from build123d import *

# Parameters (mm, degrees)
F0_W     = 19.05
F0_H     = 177.8
F1_DEPTH = 19.05
F2_R     = 3.175
F3_DEPTH = 25.4
F4_R     = 3.175
F5_DEPTH = 25.4


with BuildPart() as f1:
    # F0 (on Top) → F1 (new body, symmetric)
    with BuildSketch(Plane.XY):
        Polygon((342.9, 107.95), (-342.9, 107.95), (-342.9, 88.9), (-304.8, 88.9), (-285.75, 88.9), (-107.95, 88.9), (-88.9, 88.9), (88.9, 88.9), (107.95, 88.9), (285.75, 88.9), (304.8, 88.9), (342.9, 88.9), align=None)
        with Locations((-295.275, 0)):
            Rectangle(F0_W, F0_H)
        with Locations((295.275, 0)):
            Rectangle(F0_W, F0_H)
        Polygon((-285.75, -88.9), (-304.8, -88.9), (-342.9, -88.9), (-342.9, -107.95), (342.9, -107.95), (342.9, -88.9), (304.8, -88.9), (285.75, -88.9), (107.95, -88.9), (88.9, -88.9), (-88.9, -88.9), (-107.95, -88.9), align=None)
        with Locations((-98.425, 0)):
            Rectangle(F0_W, F0_H)
        with Locations((98.425, 0)):
            Rectangle(F0_W, F0_H)
    extrude(amount=F1_DEPTH, both=True)

    # F2 (on face) → F3 (cut)
    with BuildSketch(Plane(origin=(-304.8, 0, 0), x_dir=(0, -1, 0), z_dir=(-1, 0, 0))):
        Circle(F2_R)
    extrude(amount=-F3_DEPTH, mode=Mode.SUBTRACT)

    # F4 (on face) → F5 (cut)
    with BuildSketch(Plane.YZ.offset(304.8)):
        Circle(F4_R)
    extrude(amount=-F5_DEPTH, mode=Mode.SUBTRACT)


solid = f1.part
Work out the finished part from the listing and answer in its coordinate system (mm). A direction names the side the tool comes from. Coordinates: 2 decimals unless noted, no trailing zeros. Write each loop counter-clockwise with the first axis right and the second up, starting at its lowest first coordinate (ties: lowest second). Pieces come first, ordered by that corner, then holes. Notation, with made-up numbers: M 82.25,39 L 103.25,39 A29 ccw 103.25,69 Z; hole C -38.75,-12.75 d11. An arc over 180 degrees is marked long. Use one line per item in the form item = value. Start each with the question number.
1. A tool of negligible diameter and unlimited length cuts with its end or side. For faces 4 (the face through (-324, 88.9, 0)), 5 (the face through (5, 107.95, 0)), 6 (the face through (-198, 88.9, 0)), 7 (the face through (304.8, -1, 5)), from which of +Z, -Z, +X, -X, +Y, -Y can it reach the whole face along a straight path? Write none if from no direction.
2. Straight lines are drawn through the part: probe 1 along X at (y, z) = (-11, 2); probe 2 along Z at (x, y) = (299.5, 0) (3 decimals); probe 3 along Y at (x, z) = (-225, 16). For each, find the intervals that lie inside material, in ascending order. Write a range as from..to.
3. Each of these flat-tipped pins is pushed along its axis until it touches: P1, Ø8, axis at y = -62.5, z = -10.5, coming from the +X side; P2, Ø11.5, axis at y = 30.5, z = -6, coming from the -X side; P3, Ø5, axis at y = 0, z = 0, coming from the -X side. Where does it stop, or does it pass through?
4. The part is cut by section B-B (y = 31). Give the vertices of the cut face in (x, z).
5. The part is cut by section A-A (x = 83). Give the vertices of the cut face in (y, z).
6. The part is cut by section C-C (z = 12). Give the vertices of the cut face in (x, y), plus the area to 3 significant figures.
7. The mould has two halves that part along X. Classify faces 1 (the face through (285.75, -1, 5)), 2 (the face through (-342.9, -98, 0)), 3 (the face through (-324, -88.9, 0)): released by +X, released by -X, zero draft, split by the parting line, or undercut.
Evaluation:
q1.face_4 = +Z, -Z, -X
q1.face_5 = +Z, -Z, +X, -X, +Y
q1.face_6 = +Z, -Z
q1.face_7 = +Z, -Z, +X
q2.probe_1 = -304.8..-285.75, -107.95..-88.9, 88.9..107.95, 285.75..304.8
q2.probe_2 = -19.05..-3.175, 3.175..19.05
q2.probe_3 = -107.95..-88.9, 88.9..107.95
q3.P1 = 304.8
q3.P2 = -304.8
q3.P3 = -107.95
q4.outline = M -304.8,-19.05 L -285.75,-19.05 L -285.75,19.05 L -304.8,19.05 Z; M -107.95,-19.05 L -88.9,-19.05 L -88.9,19.05 L -107.95,19.05 Z; M 88.9,-19.05 L 107.95,-19.05 L 107.95,19.05 L 88.9,19.05 Z; M 285.75,-19.05 L 304.8,-19.05 L 304.8,19.05 L 285.75,19.05 Z
q5.outline = M -107.95,-19.05 L -88.9,-19.05 L -88.9,19.05 L -107.95,19.05 Z; M 88.9,-19.05 L 107.95,-19.05 L 107.95,19.05 L 88.9,19.05 Z
q6.outline = M -342.9,-107.95 L 342.9,-107.95 L 342.9,-88.9 L 304.8,-88.9 L 304.8,88.9 L 342.9,88.9 L 342.9,107.95 L -342.9,107.95 L -342.9,88.9 L -304.8,88.9 L -304.8,-88.9 L -342.9,-88.9 Z; hole M -285.75,-88.9 L -107.95,-88.9 L -107.95,88.9 L -285.75,88.9 Z; hole M -88.9,-88.9 L 88.9,-88.9 L 88.9,88.9 L -88.9,88.9 Z; hole M 107.95,-88.9 L 285.75,-88.9 L 285.75,88.9 L 107.95,88.9 Z
q6.area = 39,700 mm^2
q7.face_1 = undercut
q7.face_2 = released by -X
q7.face_3 = zero draft
